For this review, use the dimensioned drawing (mm, ordinates from the lowest corner) and the shaded views. Round coordinates to 2 decimals unless told otherwise and drop trailing zeros. Write each loop counter-clockwise with the first axis right and the second up, starting at its lowest first coordinate (ties: lowest second). Pieces come first, ordered by that corner, then holes. Notation, with made-up numbers: M -10,37.25 L 21,37.25 A27 cw 21,54.25 Z; hole C -22,-22.5 d11. An arc over 180 degrees is marked long. One line per question, with ' | ' between items.
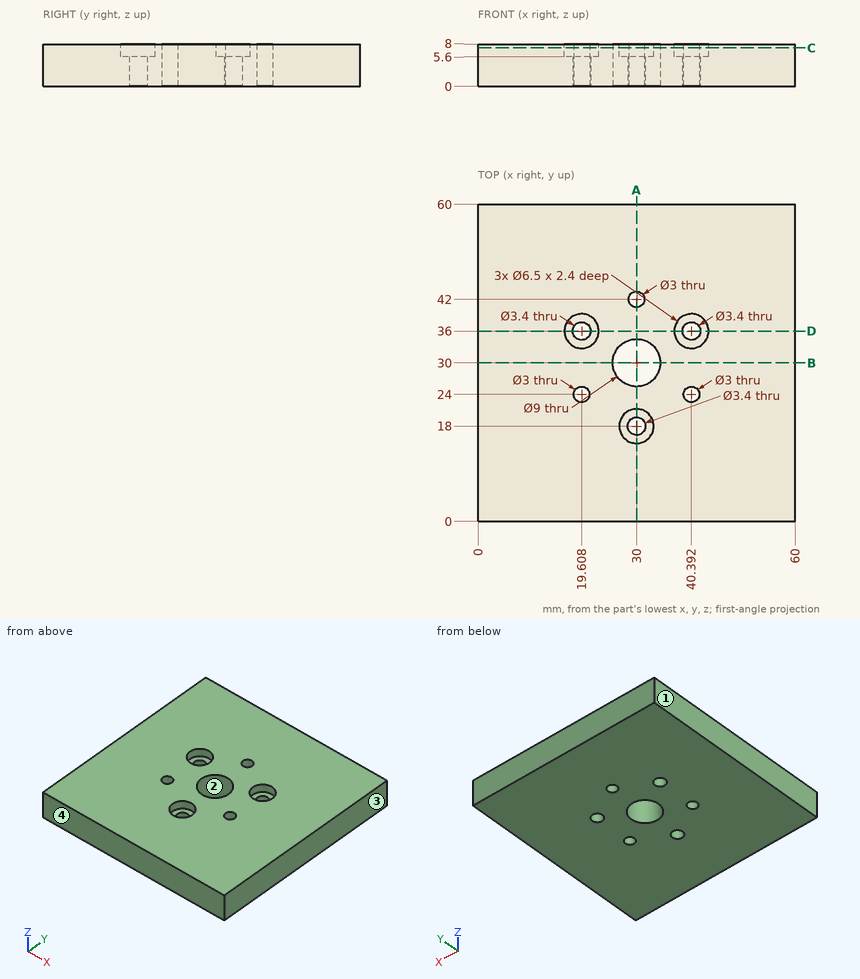
Item 1: Mouldability with a two-part tool opening along X and no side actions: class the marked faces 1, 2, 3 and 4 as +X half, -X half, draft (parallel to the pull), parting line (faces both ways), or undercut.
Results:
face 1: -X half | face 2: undercut | face 3: +X half | face 4: draft
Item 2: Insertion check: pin 1 Ø6 at (x, y) = (30, 18) entering from +Z. The pin has a flat end and moves straight along its axis. Give the tip position at first contact, or say it passes through.
Results:
pin 1: z = 5.6
Item 3: To check wall thickness, follow line 1 along Y through (x, z) = (30, 6.9); line 2 along Y through (x, z) = (30, 2.75); line 3 along X through (y, z) = (36.5, 2.25). State the ranges of each line that lie inside material, in increasing order. Write a range as from..to.
Results:
line 1: 0..14.75, 21.25..25.5, 34.5..40.5, 43.5..60 | line 2: 0..16.3, 19.7..25.5, 34.5..40.5, 43.5..60 | line 3: 0..17.98, 21.23..38.77, 42.02..60
Item 4: Take a section at A-A (x = 30). Write out the cut boundary in (y, z), then the cut area to 3 significant figures.
Results:
outline: M 0,0 L 16.3,0 L 16.3,5.6 L 14.75,5.6 L 14.75,8 L 0,8 Z; M 19.7,0 L 25.5,0 L 25.5,8 L 21.25,8 L 21.25,5.6 L 19.7,5.6 Z; M 34.5,0 L 40.5,0 L 40.5,8 L 34.5,8 Z; M 43.5,0 L 60,0 L 60,8 L 43.5,8 Z | area: 349 mm2
Item 5: Take a section at C-C (z = 7.25). Write out the cut boundary in (x, y).
Results:
outline: M 0,0 L 60,0 L 60,60 L 0,60 Z; hole C 19.61,36 d6.5; hole C 19.61,24 d3; hole C 30,30 d9; hole C 30,18 d6.5; hole C 30,42 d3; hole C 40.39,36 d6.5; hole C 40.39,24 d3
Item 6: Take a section at D-D (y = 36). Write out the cut boundary in (x, z).
Results:
outline: M 0,0 L 17.91,0 L 17.91,5.6 L 16.36,5.6 L 16.36,8 L 0,8 Z; M 21.31,0 L 38.69,0 L 38.69,5.6 L 37.14,5.6 L 37.14,8 L 22.86,8 L 22.86,5.6 L 21.31,5.6 Z; M 42.09,0 L 60,0 L 60,8 L 43.64,8 L 43.64,5.6 L 42.09,5.6 Z
Item 7: Take a section at B-B (y = 30). Write out the cut boundary in (x, z), then the cut area to 3 significant figures.
Results:
outline: M 0,0 L 25.5,0 L 25.5,8 L 0,8 Z; M 34.5,0 L 60,0 L 60,8 L 34.5,8 Z | area: 408 mm2
